```python
from build123d import *

# Parameters (mm, degrees)
F1_DEPTH = 3.81


with BuildPart() as f1:
    # F0 (on Front) → F1 (new body, symmetric)
    with BuildSketch(Plane.XZ):
        with BuildLine():
            Line((39.999735067, -7.4482769705), (1.4772535285, 18.6058512943))
            add(Edge.make_bspline(
                [(1.4772535285, 18.6058512943), (-95.952662812, -9.8829154217), (-1.8328876207, -50.3882795617)],
                knots=[3.3919385935, 3.3919385935, 3.3919385935, 5.9232263676, 5.9232263676, 5.9232263676], degree=2, weights=[1, 0.3004385759, 1]))
            Line((-1.8328876207, -50.3882795617), (39.9715108869, -25.6507564336))
            Line((39.9715108869, -25.6507564336), (46.9909198582, -25.6507564336))
            Line((46.9909198582, -25.6507564336), (46.9909198582, -7.4482769705))
            Line((46.9909198582, -7.4482769705), (39.999735067, -7.4482769705))
        make_face()
    extrude(amount=F1_DEPTH, both=True)


solid = f1.part
```
The model under review builds one solid part; all positions refer to its coordinate system, in mm. A direction names the side the tool comes from. Round coordinates to 2 decimals unless told otherwise and drop trailing zeros. Write each loop counter-clockwise with the first axis right and the second up, starting at its lowest first coordinate (ties: lowest second). Pieces come first, ordered by that corner, then holes.
(1) Wall thickness on L1, parallel to Z at x = 42, y = 3.25; L2, parallel to Z at x = 7, y = 2; L3, parallel to X at y = 2, z = 0: over which ranges is each line inside the solid? List them lowest first.
(2) We need section A-A on x = 12.5. Give the boundary of the cut face in (y, z), and give its area (3 significant figures).
(3) Machinability: for faces 1 (the flat face through (46.991, 0, -17)), 2 (the flat face through (44, 0, -7.448)), 3 (the flat face through (43, 0, -25.651)), which of the approach directions +Z, -Z, +X, -X, +Y, -Y give a long, thin tool a straight path to every point of the face, cutting with its end or side? Answer none if there is none.
(4) We need section B-B on x = 33.5. Give the boundary of the cut face in (y, z).
(5) Insertion check: pin 1 (3 mm diameter, centred on x = 10.5, y = -1, fed in from -Z); pin 2 (4 mm diameter, centred on y = -1.5, z = 6.5, fed in from -X). Each pin has a flat end and moves straight along its axis. Give the tip position at first contact, or say it passes through.
Findings below:
1. L1: z = -25.65 to -7.45
1. L2: z = -45.16 to 14.87
1. L3: x = -18.88 to 28.99
2. outline: (-3.81, -41.91) - (3.81, -41.91) - (3.81, 11.15) - (-3.81, 11.15) - close
2. area: 404 mm2
3. face 1: +Z, -Z, +X, +Y, -Y
3. face 2: +Z, +X, +Y, -Y
3. face 3: -Z, +X, +Y, -Y
4. outline: (-3.81, -29.48) - (3.81, -29.48) - (3.81, -3.05) - (-3.81, -3.05) - close
5. pin 1: stops at z = -43.98
5. pin 2: stops at x = -16.49
